Check sheet for the drawn part. Datum: minimum x, y, z corner. Units: mm. Give positions to 0.01 mm unless a question says otherwise; leave off trailing zeros. Write each loop counter-clockwise with the first axis right and the second up, starting at its lowest first coordinate (ties: lowest second). Pieces come first, ordered by that corner, then holes. Notation, with made-up numbers: M 72,-5 L 81,-5 A32 ccw 81,32 Z; hole C -38,76.5 d2. An arc over 180 degrees is marked long. Write item = value, one per line. Start each with the question number.
1) Sectioned sample at D-D, the plane x = 111.5. Record the cut outline in (y, z).
2) Gauge pin test, flat ends, axial feed: pin 1 (1.5 mm diameter, centred on x = 108.5, z = 2.5, fed in from -Y); pin 2 (1.5 mm diameter, centred on x = 7.5, z = 2.5, fed in from +Y); pin 3 (2.5 mm diameter, centred on x = 6.5, z = 1.5, fed in from -Y). Record the tip position at first contact, or that the pin passes through.
3) Sectioned sample at A-A, the plane x = 23. Record the cut outline in (y, z), then the cut area to 3 significant figures.
4) Scan lines: L1, parallel to X at y = 73.5, z = 2.95; L2, parallel to X at y = 53, z = 3.05; L3, parallel to X at y = 32, z = 4.7. Record each from-to range of solid material in increasing order.
5) Sectioned sample at B-B, the plane y = 24. Record the cut outline in (x, z).
6) Sectioned sample at C-C, the plane z = 2.7. Count the separate pieces of the cut face and the enclosed holes in it, then the cut area to 3 significant figures.
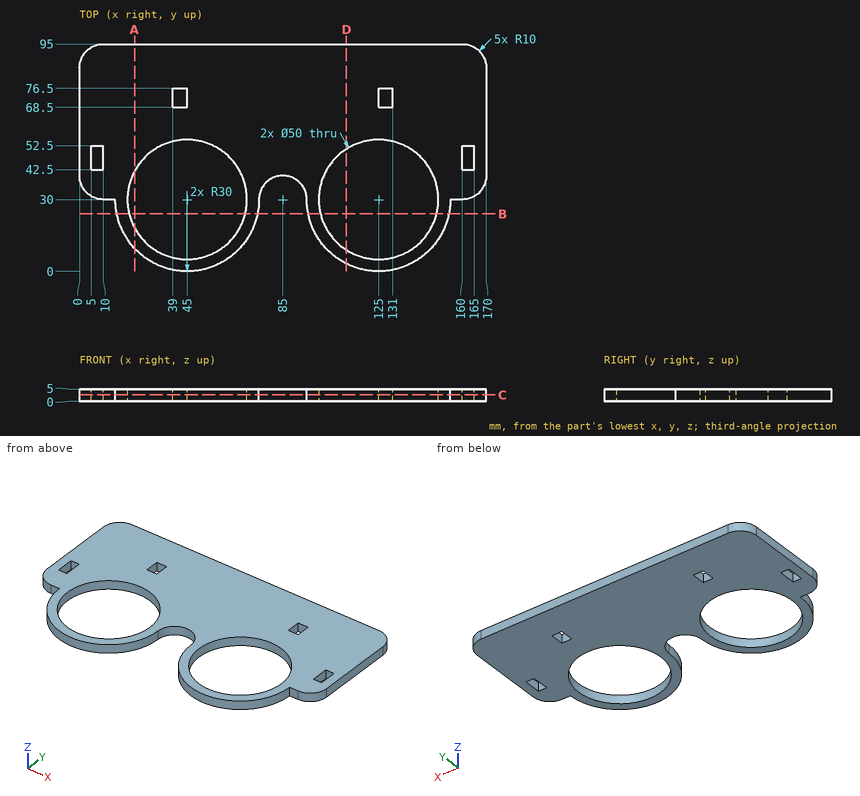
Data:
q1.outline = M 3.21,0 L 8.96,0 L 8.96,5 L 3.21,5 Z; M 51.04,0 L 95,0 L 95,5 L 51.04,5 Z
q2.pin_1 = 4.47
q2.pin_2 = 94.85
q2.pin_3 = 30.26
q3.outline = M 9.6,0 L 18.13,0 L 18.13,5 L 9.6,5 Z; M 41.87,0 L 95,0 L 95,5 L 41.87,5 Z
q3.area = 308 mm2
q4.L1 = 0 to 39, 45 to 125, 131 to 170
q4.L2 = 0 to 35.2, 54.8 to 115.2, 134.8 to 170
q4.L3 = 4 to 20.08, 69.92 to 75.2, 94.8 to 100.08, 149.92 to 166
q5.outline = M 15.61,0 L 20.73,0 L 20.73,5 L 15.61,5 Z; M 69.27,0 L 74.39,0 L 74.39,5 L 69.27,5 Z; M 95.61,0 L 100.73,0 L 100.73,5 L 95.61,5 Z; M 149.27,0 L 154.39,0 L 154.39,5 L 149.27,5 Z
q6.separate_pieces = 1
q6.enclosed_holes = 6
q6.area = 9,510 mm2
